Build history of the part. All positions in model axes, mm. A direction names the side the tool comes from. Round coordinates to 2 decimals unless told otherwise and drop trailing zeros. Write each loop counter-clockwise with the first axis right and the second up, starting at its lowest first coordinate (ties: lowest second). Pieces come first, ordered by that corner, then holes. Notation, with made-up numbers: (-17.75, 16) -> (-3.75, 16) arc R15 ccw to (-3.75, 36) -> close; hole circle Ø11 at (28.25, 34.5). An arc over 180 degrees is marked (long way). Answer as CSV lines item,"result".
from build123d import *

# Parameters (mm, degrees)
SALIENTE_EXTRUIR1_DEPTH = 90
CORTAR_EXTRUIR1_REACH   = 103.612
CROQUIS2_R              = 5


with BuildPart() as part:
    # Croquis1 → Saliente-Extruir1 (new body)
    with BuildSketch(Plane(origin=(0, 0, 0), x_dir=(0, 0, -1), z_dir=(1, 0, 0))):
        Polygon((-40, 0), (-20, 0), (-20, 6), (20, 6), (20, 0), (40, 0), (40, 25), (-40, 25), align=None)
    extrude(amount=SALIENTE_EXTRUIR1_DEPTH)

    # Croquis2 → Cortar-Extruir1 (cut, up to next)
    with BuildSketch(Plane(origin=(0, 25, 0), x_dir=(1, 0, 0), z_dir=(0, 1, 0)), mode=Mode.PRIVATE) as cortar_extruir1_sk1:
        with Locations(Location((80, -30, 0), (0, 0, 270))):
            Circle(CROQUIS2_R)
    cortar_extruir1_tool1 = extrude(cortar_extruir1_sk1.sketch, amount=-CORTAR_EXTRUIR1_REACH, mode=Mode.PRIVATE) & part.part
    # Croquis2 → Cortar-Extruir1 (cut, up to next)
    with BuildSketch(Plane(origin=(0, 25, 0), x_dir=(1, 0, 0), z_dir=(0, 1, 0)), mode=Mode.PRIVATE) as cortar_extruir1_sk2:
        with Locations(Location((10, -30, 0), (0, 0, 270))):
            Circle(CROQUIS2_R)
    cortar_extruir1_tool2 = extrude(cortar_extruir1_sk2.sketch, amount=-CORTAR_EXTRUIR1_REACH, mode=Mode.PRIVATE) & part.part
    # Croquis2 → Cortar-Extruir1 (cut, up to next)
    with BuildSketch(Plane(origin=(0, 25, 0), x_dir=(1, 0, 0), z_dir=(0, 1, 0)), mode=Mode.PRIVATE) as cortar_extruir1_sk3:
        with Locations(Location((80, 30, 0), (0, 0, 270))):
            Circle(CROQUIS2_R)
    cortar_extruir1_tool3 = extrude(cortar_extruir1_sk3.sketch, amount=-CORTAR_EXTRUIR1_REACH, mode=Mode.PRIVATE) & part.part
    # Croquis2 → Cortar-Extruir1 (cut, up to next)
    with BuildSketch(Plane(origin=(0, 25, 0), x_dir=(1, 0, 0), z_dir=(0, 1, 0)), mode=Mode.PRIVATE) as cortar_extruir1_sk4:
        with Locations(Location((10, 30, 0), (0, 0, 270))):
            Circle(CROQUIS2_R)
    cortar_extruir1_tool4 = extrude(cortar_extruir1_sk4.sketch, amount=-CORTAR_EXTRUIR1_REACH, mode=Mode.PRIVATE) & part.part
    add(cortar_extruir1_tool1.solids().sort_by_distance((80, 25, 30))[0], mode=Mode.SUBTRACT)
    add(cortar_extruir1_tool2.solids().sort_by_distance((10, 25, 30))[0], mode=Mode.SUBTRACT)
    add(cortar_extruir1_tool3.solids().sort_by_distance((80, 25, -30))[0], mode=Mode.SUBTRACT)
    add(cortar_extruir1_tool4.solids().sort_by_distance((10, 25, -30))[0], mode=Mode.SUBTRACT)

    # Croquis4 → Recubrir4 section 0
    with BuildSketch(Plane.XY.offset(40)):
        with BuildLine():
            Line((17.5, 25), (42.5, 25))
            ThreePointArc((42.5, 25), (30, 37.5), (17.5, 25))
        make_face()
    # Croquis3 → Recubrir4 section 1
    with BuildSketch(Plane(origin=(0, 0, -40), x_dir=(-1, 0, 0), z_dir=(0, 0, -1))):
        with BuildLine():
            Line((-72.5, 25), (-47.5, 25))
            ThreePointArc((-47.5, 25), (-60, 37.5), (-72.5, 25))
        make_face()
    loft()

    # Cortar-Recubrir1: read off the stored shape, not the designer's step
    # Cortar-Recubrir1: loft between two sections, ruled curve by curve
    cortar_recubrir1_from = [
        Edge.make_bspline([(66.474673977, 28.785313314, -40), (66.159231201, 29.324869479, -40), (65.736792303, 29.896857571, -40), (64.865302784, 30.721785457, -40), (64.535116198, 30.990385277, -40), (63.787281531, 31.48910574, -40), (63.369421529, 31.719151625, -40), (62.447680858, 32.106958451, -40), (61.943610916, 32.26447662, -40), (60.867132061, 32.469827705, -40), (60.294709068, 32.517257966, -40), (59.119137062, 32.471285113, -40), (58.516285627, 32.377485336, -40), (57.333561907, 32.036960006, -40), (56.754242851, 31.790116754, -40), (55.675130521, 31.159231201, -40), (55.17584807, 30.775487545, -40), (54.298935855, 29.911880072, -40), (53.921474907, 29.432556086, -40), (53.304749619, 28.430691343, -40), (53.065285592, 27.908604481, -40), (52.716177882, 26.869807291, -40), (52.606176412, 26.353282213, -40), (52.491969247, 25.359825257, -40), (52.487459152, 24.882847533, -40), (52.555211917, 23.986528197, -40), (52.627305677, 23.567038585, -40), (52.918664408, 22.402946626, -40), (53.209883246, 21.754242851, -40), (53.840768799, 20.675130521, -40), (54.263207697, 20.103142429, -40), (55.134697216, 19.278214543, -40), (55.464883802, 19.009614723, -40), (56.212718469, 18.51089426, -40), (56.630578471, 18.280848375, -40), (57.552319142, 17.893041549, -40), (58.056389084, 17.73552338, -40), (59.132867939, 17.530172295, -40), (59.705290932, 17.482742034, -40), (60.880862938, 17.528714887, -40), (61.483714373, 17.622514664, -40), (62.666438093, 17.963039994, -40), (63.245757149, 18.209883246, -40), (64.324869479, 18.840768799, -40), (64.82415193, 19.224512455, -40), (65.701064145, 20.088119928, -40), (66.078525093, 20.567443914, -40), (66.695250381, 21.569308657, -40), (66.934714408, 22.091395519, -40), (67.283822118, 23.130192709, -40), (67.393823588, 23.646717787, -40), (67.508030753, 24.640174743, -40), (67.512540848, 25.117152467, -40), (67.444788083, 26.013471803, -40), (67.372694323, 26.432961415, -40), (67.081335592, 27.597053374, -40), (66.790116754, 28.245757149, -40), (66.474673977, 28.785313314, -40)], [0, 0, 0, 0, 0.0625, 0.0625, 0.09375, 0.09375, 0.125, 0.125, 0.15625, 0.15625, 0.1875, 0.1875, 0.21875, 0.21875, 0.25, 0.25, 0.28125, 0.28125, 0.3125, 0.3125, 0.34375, 0.34375, 0.375, 0.375, 0.40625, 0.40625, 0.4375, 0.4375, 0.5, 0.5, 0.5625, 0.5625, 0.59375, 0.59375, 0.625, 0.625, 0.65625, 0.65625, 0.6875, 0.6875, 0.71875, 0.71875, 0.75, 0.75, 0.78125, 0.78125, 0.8125, 0.8125, 0.84375, 0.84375, 0.875, 0.875, 0.90625, 0.90625, 0.9375, 0.9375, 1, 1, 1, 1], 3),
    ]
    cortar_recubrir1_to = [
        Edge.make_bspline([(29.971725733, 32.499946704, 40), (29.346730174, 32.497590515, 40), (28.640021711, 32.418925734, 40), (27.489296584, 32.078585195, 40), (27.091335491, 31.927601711, 40), (26.284847367, 31.530668849, 40), (25.876278751, 31.284498632, 40), (25.078546377, 30.681486974, 40), (24.689497752, 30.324360039, 40), (23.972030096, 29.495978512, 40), (23.643952375, 29.024509827, 40), (23.094236484, 27.984367777, 40), (22.873090724, 27.415752966, 40), (22.574631411, 26.22171991, 40), (22.497697107, 25.596721292, 40), (22.502409485, 24.346730174, 40), (22.584053936, 23.722329387, 40), (22.891507477, 22.53058058, 40), (23.116934166, 21.963649315, 40), (23.674476843, 20.927681551, 40), (24.006099995, 20.458699891, 40), (24.729793048, 19.635751438, 40), (25.121523263, 19.281567984, 40), (25.923779519, 18.684588169, 40), (26.334192585, 18.441505455, 40), (27.143650559, 18.050664595, 40), (27.542738719, 17.902685931, 40), (28.69599722, 17.571031246, 40), (29.403278708, 17.497697107, 40), (30.653269826, 17.502409485, 40), (31.359978289, 17.581074266, 40), (32.510703416, 17.921414805, 40), (32.908664509, 18.072398289, 40), (33.715152633, 18.469331151, 40), (34.123721249, 18.715501368, 40), (34.921453623, 19.318513026, 40), (35.310502248, 19.675639961, 40), (36.027969904, 20.504021488, 40), (36.356047625, 20.975490173, 40), (36.905763516, 22.015632223, 40), (37.126909276, 22.584247034, 40), (37.425368589, 23.77828009, 40), (37.502302893, 24.403278708, 40), (37.497590515, 25.653269826, 40), (37.415946064, 26.277670613, 40), (37.108492523, 27.46941942, 40), (36.883065834, 28.036350685, 40), (36.325523157, 29.072318449, 40), (35.993900005, 29.541300109, 40), (35.270206952, 30.364248562, 40), (34.878476737, 30.718432016, 40), (34.076220481, 31.315411831, 40), (33.665807415, 31.558494545, 40), (32.856349441, 31.949335405, 40), (32.457261281, 32.097314069, 40), (31.30400278, 32.428968754, 40), (30.596721292, 32.502302893, 40), (29.971725733, 32.499946704, 40)], [0, 0, 0, 0, 0.0625, 0.0625, 0.09375, 0.09375, 0.125, 0.125, 0.15625, 0.15625, 0.1875, 0.1875, 0.21875, 0.21875, 0.25, 0.25, 0.28125, 0.28125, 0.3125, 0.3125, 0.34375, 0.34375, 0.375, 0.375, 0.40625, 0.40625, 0.4375, 0.4375, 0.5, 0.5, 0.5625, 0.5625, 0.59375, 0.59375, 0.625, 0.625, 0.65625, 0.65625, 0.6875, 0.6875, 0.71875, 0.71875, 0.75, 0.75, 0.78125, 0.78125, 0.8125, 0.8125, 0.84375, 0.84375, 0.875, 0.875, 0.90625, 0.90625, 0.9375, 0.9375, 1, 1, 1, 1], 3),
    ]
    cortar_recubrir1 = Solid(Shell([*[Face.make_surface_from_curves(cortar_recubrir1_from[k], cortar_recubrir1_to[k]) for k in range(1)], Face(Wire(cortar_recubrir1_from)), Face(Wire(cortar_recubrir1_to))]))
    add(cortar_recubrir1, mode=Mode.SUBTRACT)


solid = part.part
1. Mould opens along X. For faces 6 (the flat face through (44, 3, -20)), 7 (the flat face through (0, 13, 1)), 8 (the cylindrical face through (10, 13, -35)) say: +X half, -X half, draft (parallel to the pull), parting line (faces both ways), or undercut.
Results found:
face 6,"draft"
face 7,"-X half"
face 8,"undercut"
2. Cut at A-A, the plane y = 4. Write the cut outline in (x, z).
Results found:
outline,"(0, -40) -> (90, -40) -> (90, -20) -> (0, -20) -> close; (0, 20) -> (90, 20) -> (90, 40) -> (0, 40) -> close; hole circle Ø10 at (10, -30); hole circle Ø10 at (10, 30); hole circle Ø10 at (80, -30); hole circle Ø10 at (80, 30)"
3. Probe line 1 along X through (y, z) = (9, 30); line 2 along Z through (x, y) = (6, 4); line 3 along X through (y, z) = (19, 30). List the from-to ranges inside material, lowest first.
Results found:
line 1,"x = 0 to 5, 15 to 75, 85 to 90"
line 2,"z = -40 to -33, -27 to -20, 20 to 27, 33 to 40"
line 3,"x = 0 to 5, 15 to 29.99, 37.51 to 75, 85 to 90"
4. Drop flat-ended pins along their axis: pin 1 Ø20 at (x, z) = (56, 0.5) entering from -Y; pin 2 Ø9 at (x, z) = (80, -30) entering from -Y; pin 3 Ø11.5 at (x, z) = (10, 30) entering from +Y. Give the stop position or say it passes through.
Results found:
pin 1,"stops at y = 6"
pin 2,"passes through"
pin 3,"stops at y = 25"
5. Which spindle directions (+Z, -Z, +X, -X, +Y, -Y) get a long thin tool onto all of the face, cutting with end or side? Do faces 1 (the flat face through (90, 13, 1)), 2 (the flat face through (18, 25, -9)), 3 (the flat face through (71, 25, 8)), 4 (the flat face through (44, 6, 0)), 5 (the flat face through (44, 0, 30)). Say none if no direction does.
Results found:
face 1,"+Z, -Z, +X, +Y, -Y"
face 2,"-Z, -X, +Y"
face 3,"+Z, +X, +Y"
face 4,"+X, -X, -Y"
face 5,"+Z, -Z, +X, -X, -Y"
6. Cut at B-B, the plane x = 82. Write the cut outline in (y, z).
Results found:
outline,"(0, -40) -> (25, -40) -> (25, -34.58) -> (0, -34.58) -> close; (0, -25.42) -> (25, -25.42) -> (25, 25.42) -> (0, 25.42) -> (0, 20) -> (6, 20) -> (6, -20) -> (0, -20) -> close; (0, 34.58) -> (25, 34.58) -> (25, 40) -> (0, 40) -> close"
7. Cut at C-C, the plane z = -30. Count the separate pieces of the cut face and the enclosed holes in it, then the cut area to 3 significant figures.
Results found:
separate pieces,"3"
enclosed holes,"1"
area,"1,840 mm2"
